Part model, mm, in its own coordinate system. Face numbers are marked on the shaded views. A direction names the side the tool comes from. Round coordinates to 2 decimals unless told otherwise and drop trailing zeros. Order: outer loops, then holes, each group sorted by start corner. A loop starts at its lowest first (then second) coordinate and runs counter-clockwise, first axis right, second up. Notation, with made-up numbers: (-13.5, 22.25) - (17.5, 22.25) arc R16 ccw to (17.5, 26.25) - close; hole circle Ø4 at (23, 53.25). An arc over 180 degrees is marked (long way). Answer as a JSON object with one key per item and string values.
```python
from build123d import *

# Parameters (mm, degrees)
F1_DEPTH = 50
F2_W     = 88.2
F2_H     = 38.2
F2_W_2   = 43.121268
F2_H_2   = 15.88
F3_DEPTH = 25
F4_SIZE2 = 11.547005
F4_SIZE  = 20


with BuildPart() as f1:
    # F0 (on Top) → F1 (new body)
    with BuildSketch(Plane.XY):
        Polygon((50, 218.464008), (0, 218.464008), (-50, 218.464008), (-66.227116, 190.357819), (-66.227116, 161.646203), (-66.227116, 0), (-66.227116, -59.276793), (-66.227116, -208.420123), (-53.694672, -208.420123), (-53.694672, -59.276793), (0, -59.276793), (53.694672, -59.276793), (53.694672, -208.420123), (66.227116, -208.420123), (66.227116, -59.276793), (66.227116, 0), (66.227116, 161.646203), (66.227116, 190.357819), align=None)
        Polygon((-66.227116, 0), (-66.227116, 161.646203), (-96.047964, 161.646203), (-127.75892, 116.358264), (-127.75892, 86.03783), (-127.75892, -49.467381), (-127.75892, -59.276793), (-66.227116, -59.276793), align=None)
        Polygon((-127.75892, -49.467381), (-127.75892, 86.03783), (-169.235751, 44.560999), (-169.235751, -49.467381), align=None)
        Polygon((96.047964, 161.646203), (66.227116, 161.646203), (66.227116, 0), (66.227116, -59.276793), (127.75892, -59.276793), (127.75892, -49.467381), (127.75892, 86.03783), (127.75892, 116.358264), align=None)
        Polygon((169.235751, 44.560999), (127.75892, 86.03783), (127.75892, -49.467381), (169.235751, -49.467381), align=None)
    extrude(amount=-F1_DEPTH)

    # F2 (on face) → F3 (join)
    with BuildSketch(Plane(origin=(0, 218.464008, 0), x_dir=(-1, 0, 0), z_dir=(0, 1, 0))):
        with Locations((0, -25)):
            Rectangle(F2_W, F2_H)
        with Locations((0, -25)):
            Rectangle(F2_W_2, F2_H_2, mode=Mode.SUBTRACT)
        with Locations((0, -25)):
            Rectangle(F2_W_2, F2_H_2)
    extrude(amount=F3_DEPTH)

    # F4
    f4_edges = [f1.edges().sort_by_distance(p)[0] for p in [
        (-44.1, 243.464008, -25),
        (0, 243.464008, -5.9),
        (44.1, 243.464008, -25),
        (0, 243.464008, -44.1),
    ]]
    chamfer(f4_edges, length=F4_SIZE, length2=F4_SIZE2)


solid = f1.part
```
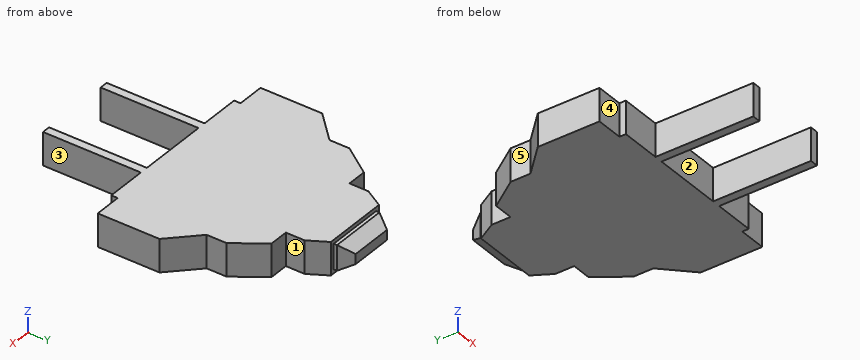
Item 1: Probe L1, parallel to X at y = -149, z = -39.5; L2, parallel to Y at x = -147.5, z = -30; L3, parallel to Y at x = -4.5, z = -23.5. List the from-to ranges inside material, lowest first. Write a range as from..to.
Taken from the geometry:
{"L1": "-66.23..-53.69, 53.69..66.23", "L2": "-49.47..66.3", "L3": "-59.28..243.46"}
Item 2: Tool access for the marked faces 1, 2, 3, 4 and 5: list every direction of +Z, -Z, +X, -X, +Y, -Y with a clear straight run to the whole face (end or side of a thin tool).
Taken from the geometry:
{"face 1": "+Z, -Z, +X, +Y", "face 2": "+Z, -Z, -Y", "face 3": "+Z, -Z, +X, -Y", "face 4": "+Z, -Z, -X, -Y", "face 5": "+Z, -Z, -X, +Y"}
Item 3: Cut at A-A (y = -126). Write the cut outline in (x, z), plus the area to 3 significant figures.
Taken from the geometry:
{"outline": "(-66.23, -50) - (-53.69, -50) - (-53.69, 0) - (-66.23, 0) - close; (53.69, -50) - (66.23, -50) - (66.23, 0) - (53.69, 0) - close", "area": "1,250 mm2"}
Item 4: Cut at C-C (x = -24). Write the cut outline in (y, z).
Taken from the geometry:
{"outline": "(-59.28, -50) - (218.46, -50) - (218.46, -44.1) - (223.46, -44.1) - (243.46, -32.55) - (243.46, -17.45) - (223.46, -5.9) - (218.46, -5.9) - (218.46, 0) - (-59.28, 0) - close"}
Item 5: Cut at D-D (y = 91.5). Write the cut outline in (x, z).
Taken from the geometry:
{"outline": "(-127.76, -50) - (127.76, -50) - (127.76, 0) - (-127.76, 0) - close"}
Item 6: Drop flat-ended pins along their axis: P1, Ø9, axis at x = 86, z = -13, coming from the +Y side; P2, Ø1.5, axis at x = 10, y = 221, coming from the -Z side; P3, Ø23, axis at y = 176, z = -16.5, coming from the -X side; P4, Ø12, axis at x = 108.5, y = 120.5, coming from the +Z side. Give the stop position or say it passes through.
Taken from the geometry:
{"P1": "y = 161.65", "P2": "z = -44.1", "P3": "x = -66.23", "P4": "z = 0"}
